Part model, mm, in its own coordinate system. Give positions to 0.01 mm unless a question says otherwise; leave off trailing zeros. Write each loop counter-clockwise with the first axis right and the second up, starting at its lowest first coordinate (ties: lowest second). Pieces come first, ordered by that corner, then holes. Notation, with made-up numbers: M 89,-17 L 136,-17 A20 cw 136,-5 Z; hole C 87.25,60.5 d7. An arc over 180 degrees is marked long. Use a Markdown table: item, result.
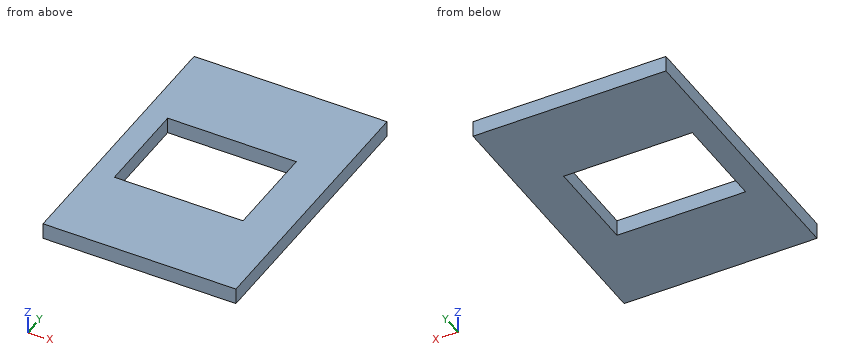
Autodesk Fusion 360 part; units mm, degrees
sketch "Sketch1" plane through (0, 0, 0) normal (0, 0, 1) x (1, 0, 0)
  line L0 (0, 0) -> (60, 0)
  line L1 (60, 0) -> (60, -85)
  line L2 (60, -85) -> (0, -85)
  line L3 (0, -85) -> (0, 0)
  line L4 (7, -27.5) -> (47, -27.5)
  line L5 (47, -27.5) -> (47, -57.5)
  line L6 (47, -57.5) -> (7, -57.5)
  line L7 (7, -57.5) -> (7, -27.5)
  dimension "d7" = 60
  dimension "d8" = 85
  dimension "d15" = 40
  dimension "d16" = 30
  dimension "d17" = 7
  dimension "d18" = 27.5
extrude "Extrude1" add sketch "Sketch1" along normal blind 5 contours L0 L1 L2 L3 | L4 L5 L6 L7
extrude "Extrude2" cut sketch "Sketch1" along normal blind 100 contours L4 L5 L6 L7
equation "perfboard_length = 65 mm"
equation "perfboard_width = 40 mm"
equation "width = perfboard_length + 2 * screw_radius * 2"
equation "length = perfboard_width + 2 * screw_radius * 2"
equation "height = 5 mm"
equation "d7 = length"
equation "d8 = width"
equation "d9 = height"
equation "middle_gap_width = 30 mm"
equation "middle_gap_length = length - 2 * screw_radius * 2"
equation "middle_gap_small_distance = 7 mm"
equation "middle_gap_big_distance = ( width - middle_gap_width ) / 2"
equation "d15 = middle_gap_length"
equation "d16 = middle_gap_width"
equation "d17 = middle_gap_small_distance"
equation "d18 = middle_gap_big_distance"
equation "extra = 100 mm"
equation "d20 = extra"
equation "screw_radius = 5 mm"
1. Cut at C-C, the plane z = 2.85. Give the cut face in (x, y), then the cut area to 3 significant figures.
Findings below:
| item | result |
|---|---|
| outline | M 0,-85 L 60,-85 L 60,0 L 0,0 Z; hole M 7,-57.5 L 47,-57.5 L 47,-27.5 L 7,-27.5 Z |
| area | 3,900 mm2 |
2. Drill centre lines: L1, parallel to X at y = -37, z = 0.2; L2, parallel to Y at x = 13, z = 4.65. Where is each one in solid material? Low to high.
Findings below:
| item | result |
|---|---|
| L1 | 0 to 7, 47 to 60 |
| L2 | -85 to -57.5, -27.5 to 0 |
3. Cut at A-A, the plane y = -29.5. Give the cut face in (x, z), then the cut area to 3 significant figures.
Findings below:
| item | result |
|---|---|
| outline | M 0,0 L 7,0 L 7,5 L 0,5 Z; M 47,0 L 60,0 L 60,5 L 47,5 Z |
| area | 100 mm2 |
4. Cut at B-B, the plane x = 14. Give the cut face in (y, z).
Findings below:
| item | result |
|---|---|
| outline | M -85,0 L -57.5,0 L -57.5,5 L -85,5 Z; M -27.5,0 L 0,0 L 0,5 L -27.5,5 Z |
